Verification items for the finished model (mm, model axes). Coordinates: 2 decimals unless noted, no trailing zeros. Loops run counter-clockwise (first coordinate to the right, second up) from the corner with the lowest first, then second, coordinate; pieces in that order, holes last.
Q1. Sectioned sample at A-A (y = 0). Enter the section's corners in (x, z).
Q2. Material ranges on probe 1 along Z at (x, y) = (0.55, 2.75); probe 2 along Z at (x, y) = (0.15, 2.5); probe 3 along Z at (x, y) = (0.2, -0.5), recorded low to high.
Q3. Sectioned sample at D-D (z = 0). Enter the section's corners in (x, y), then the cut area to 3 significant figures.
Q4. Sectioned sample at B-B (y = -1). Enter the section's corners in (x, z), then the cut area to 3 significant figures.
Q5. Mould release check, pull along Z, two halves, no side actions. Record for faces 1 (the face through (0.394, 4.497, 0.155)), 2 (the face through (0, 2.3, -0.1)), 3 (the face through (0.4, 2.1, -2.8)), 4 (the face through (0.4, 2.1, 2.8)): +Z half, -Z half, draft (parallel to the pull), parting line (faces both ways), or undercut.
Q6. Sectioned sample at C-C (x = 0.5). Enter the section's corners in (y, z).
```python
from build123d import *

# Parameters (mm, degrees)
EXTRUDE_1_DEPTH = 0.8


with BuildPart() as part:
    # 草图1 → 凸台-拉伸1 (new body)
    with BuildSketch(Plane(origin=(0, 0, 0), x_dir=(0, 0, -1), z_dir=(1, 0, 0))):
        with BuildLine():
            Line((-1.622319151, -2.316911861), (-2.402867712, -3.431650734))
            ThreePointArc((-2.402867712, -3.431650734), (-2.607110405, -3.556693113), (-2.837799992, -3.492404789))
            ThreePointArc((-2.837799992, -3.492404789), (0, 4.5), (2.837799992, -3.492404789))
            ThreePointArc((2.837799992, -3.492404789), (2.607110405, -3.556693113), (2.402867712, -3.431650734))
            Line((2.402867712, -3.431650734), (1.622319151, -2.316911861))
            ThreePointArc((1.622319151, -2.316911861), (1.441481842, -1.738720971), (1.627647463, -1.162223617))
            ThreePointArc((1.627647463, -1.162223617), (1.9404922, -0.484241696), (1.982865646, 0.261235201))
            ThreePointArc((1.982865646, 0.261235201), (2.030846926, 0.467080052), (2.202649779, 0.59019823))
            Line((2.202649779, 0.59019823), (3.077349334, 0.824573269))
            ThreePointArc((3.077349334, 0.824573269), (3.266264026, 0.97670818), (3.280925835, 1.218821425))
            ThreePointArc((3.280925835, 1.218821425), (2.776736691, 2.130665002), (2.026457183, 2.853676801))
            ThreePointArc((2.026457183, 2.853676801), (1.788798992, 2.902178099), (1.592953232, 2.759075932))
            Line((1.592953232, 2.759075932), (1.140175425, 1.974841766))
            ThreePointArc((1.140175425, 1.974841766), (0.976786548, 1.840758282), (0.765537221, 1.847688492))
            ThreePointArc((0.765537221, 1.847688492), (0, 2), (-0.765537221, 1.847688492))
            ThreePointArc((-0.765537221, 1.847688492), (-0.976786548, 1.840758282), (-1.140175425, 1.974841766))
            Line((-1.140175425, 1.974841766), (-1.592953232, 2.759075932))
            ThreePointArc((-1.592953232, 2.759075932), (-1.788798992, 2.902178099), (-2.026457183, 2.853676801))
            ThreePointArc((-2.026457183, 2.853676801), (-2.776736691, 2.130665002), (-3.280925835, 1.218821425))
            ThreePointArc((-3.280925835, 1.218821425), (-3.266264026, 0.97670818), (-3.077349334, 0.824573269))
            Line((-3.077349334, 0.824573269), (-2.202649779, 0.59019823))
            ThreePointArc((-2.202649779, 0.59019823), (-2.030846926, 0.467080052), (-1.982865646, 0.261235201))
            ThreePointArc((-1.982865646, 0.261235201), (-1.9404922, -0.484241696), (-1.627647463, -1.162223617))
            ThreePointArc((-1.627647463, -1.162223617), (-1.441481842, -1.738720971), (-1.622319151, -2.316911861))
        make_face()
    extrude(amount=EXTRUDE_1_DEPTH)


solid = part.part
```
Geometry check:
1. outline: (0, -4.5) - (0.8, -4.5) - (0.8, -2) - (0, -2) - close; (0, 2) - (0.8, 2) - (0.8, 4.5) - (0, 4.5) - close
2. probe 1: z = -3.56 to -2.17, -1.59 to 1.59, 2.17 to 3.56
2. probe 2: z = -3.74 to -2.45, -1.44 to 1.44, 2.45 to 3.74
2. probe 3: z = -4.47 to -1.94, 1.94 to 4.47
3. outline: (0, 2) - (0.8, 2) - (0.8, 4.5) - (0, 4.5) - close
3. area: 2.00 mm2
4. outline: (0, -4.39) - (0.8, -4.39) - (0.8, -1.73) - (0, -1.73) - close; (0, 1.73) - (0.8, 1.73) - (0.8, 4.39) - (0, 4.39) - close
4. area: 4.25 mm2
5. face 1: parting line
5. face 2: draft
5. face 3: undercut
5. face 4: undercut
6. outline: (-3.49, -2.84) arc R4.5 ccw (long way) to (-3.49, 2.84) arc R0.3 ccw to (-3.43, 2.4) - (-2.32, 1.62) arc R1 ccw to (-1.16, 1.63) arc R2 cw to (0.26, 1.98) arc R0.3 ccw to (0.59, 2.2) - (0.82, 3.08) arc R0.3 cw to (1.22, 3.28) arc R3.5 cw to (2.85, 2.03) arc R0.3 cw to (2.76, 1.59) - (1.97, 1.14) arc R0.3 ccw to (1.85, 0.77) arc R2 cw to (1.85, -0.77) arc R0.3 ccw to (1.97, -1.14) - (2.76, -1.59) arc R0.3 cw to (2.85, -2.03) arc R3.5 cw to (1.22, -3.28) arc R0.3 cw to (0.82, -3.08) - (0.59, -2.2) arc R0.3 ccw to (0.26, -1.98) arc R2 cw to (-1.16, -1.63) arc R1 ccw to (-2.32, -1.62) - (-3.43, -2.4) arc R0.3 ccw to start
